from build123d import *

# Parameters (mm, degrees)
SKETCH1_R               = 32
BOSS_EXTRUDE1_DEPTH     = 100
SKETCH2_R               = 30.025
CUT_EXTRUDE1_DEPTH      = 59
SKETCH3_R               = 32
BOSS_EXTRUDE2_DEPTH     = 2
CUT_EXTRUDE2_DEPTH      = 4
CUT_EXTRUDE2_DEPTH_BACK = 4
SKETCH4_W               = 70.13553728
SKETCH4_H               = 5.843920962


with BuildPart() as part:
    # Sketch1 → Boss-Extrude1 (new body)
    with BuildSketch(Plane(origin=(0, 0, 0), x_dir=(1, 0, 0), z_dir=(0, 1, 0))):
        with Locations(Location((0, 0, 0), (0, 0, 270))):
            Circle(SKETCH1_R)
    extrude(amount=BOSS_EXTRUDE1_DEPTH)

    # Sketch2 → Cut-Extrude1 (cut)
    with BuildSketch(Plane.XZ):
        with Locations(Location((0, 0, 0), (0, 0, 270))):
            Circle(SKETCH2_R)
    extrude(amount=-CUT_EXTRUDE1_DEPTH, mode=Mode.SUBTRACT)

    # Sketch3 → Boss-Extrude2 (add)
    with BuildSketch(Plane(origin=(0, 100, 0), x_dir=(1, 0, 0), z_dir=(0, 1, 0))):
        with Locations(Location((0, 0, 0), (0, 0, 270))):
            Circle(SKETCH3_R)
    extrude(amount=BOSS_EXTRUDE2_DEPTH)

    # Sketch4 → Cut-Extrude2 (cut, two sides: drawn at the far end of the back side and taken through both)
    with BuildSketch(Plane.XY.offset(-CUT_EXTRUDE2_DEPTH_BACK)):
        with Locations((-0.197032679, -0.331379703)):
            Rectangle(SKETCH4_W, SKETCH4_H)
    extrude(amount=CUT_EXTRUDE2_DEPTH + CUT_EXTRUDE2_DEPTH_BACK, mode=Mode.SUBTRACT)


solid = part.part
Input: part model. Units: mm. Frame: model coordinates. A direction names the side the tool comes from. Coordinates: 2 decimals unless noted, no trailing zeros. Loops run counter-clockwise (first coordinate to the right, second up) from the corner with the lowest first, then second, coordinate; pieces in that order, holes last.
(1) Section C-C on y = 12. Return the cut outline in (x, z) (3 decimals).
(2) First-contact query: pin 1 Ø2 at (x, y) = (-30.5, 1) entering from -Z; pin 2 Ø1.6 at (x, y) = (-30.5, 1.5) entering from +Z; pin 3 Ø1.5 at (x, z) = (-4, -19) entering from -Y. Flat tips, straight axial feed; report the tip coordinate or a pass-through.
(3) Section B-B on x = 0. Return the cut outline in (y, z) (3 decimals).
(4) Section D-D on y = 75. Return the cut outline in (x, z).
(5) Material intervals for probe 1 along X at (y, z) = (30, 0) (3 decimals); probe 2 along Y at (x, z) = (-18.5, -22), sorted ascending.
(6) Set-up query: faces 4 (the face through (-29.31, 29.09, 6.51)), 5 (the face through (31, 2.591, 0)), 6 (the face through (0, 102, 0)). Return all of +Z, -Z, +X, -X, +Y, -Y with unobstructed straight access to the full face (end or side cutting, diameter ignored); none if empty.
(7) Pull-direction query (X, two-part tool) for faces 1 (the face through (0, 59, 0)), 2 (the face through (-31.24, 50.29, -6.94)), 3 (the face through (-31, 2.591, 0)); classes: released by +X, released by -X, zero draft, split by the parting line, or undercut.
(8) Section A-A on z = 0. Return the cut outline in (x, y) (3 decimals), then the cut area to 3 significant figures.
Data:
1. outline: circle Ø64 at (0, 0); hole circle Ø60.05 at (0, 0)
2. pin 1: stops at z = -12.4
2. pin 2: stops at z = 11.91
2. pin 3: stops at y = 59
3. outline: (0, -32) - (102, -32) - (102, 32) - (0, 32) - (0, 30.025) - (59, 30.025) - (59, -30.025) - (0, -30.025) - close
4. outline: circle Ø64 at (0, 0)
5. probe 1: x = -32 to -30.025, 30.025 to 32
5. probe 2: y = 59 to 102
6. face 4: -Y
6. face 5: +X, -X, -Y
6. face 6: +Z, -Z, +X, -X, +Y
7. face 1: undercut
7. face 2: split by the parting line
7. face 3: zero draft
8. outline: (-32, 2.591) - (-30.025, 2.591) - (-30.025, 59) - (30.025, 59) - (30.025, 2.591) - (32, 2.591) - (32, 102) - (-32, 102) - close
8. area: 2,970 mm2
